Read the model definition and answer for the solid it produces. Units are mm, in the model's axes. Face numbers are marked on the shaded views. A direction names the side the tool comes from. Coordinates: 2 decimals unless noted, no trailing zeros. Order: outer loops, then holes, each group sorted by start corner. A loop starts at its lowest first (then second) coordinate and runs counter-clockwise, first axis right, second up. Notation, with made-up numbers: M -8,53 L 21,53 A33 cw 21,87 Z; hole C 34,70 d5. An arc over 180 degrees is marked long. One line per question, with ' | ' between items. Start each with the question number.
1) Consider probe 1 along Z at (x, y) = (2, 25); probe 2 along X at (y, z) = (18, 20.5); probe 3 along Y at (x, z) = (22.5, 63.75). Determine where each line is inside the solid, lowest interval first.
2) Find section D-D, the plane y = 4. Write down the section's boundary in (x, z), plus the area to 3 significant figures.
3) Find section A-A, the plane z = 40. Write down the section's boundary in (x, y), plus the area to 3 significant figures.
4) A tool of negligible diameter and unlimited length cuts with its end or side. For the marked faces 5, 6 and 7, from which of +Z, -Z, +X, -X, +Y, -Y can it reach the whole face along a straight path? Write none if from no direction.
5) Given P1, Ø23, axis at y = 25, z = 40, coming from the +X side; P2, Ø5, axis at x = 50.5, y = 32, coming from the +Z side; P3, Ø24, axis at x = 22.5, y = 25, coming from the -Z side, each flat-ended and moving along its own axis, determine where each tip first touches the part or whether it passes through.
6) The mould has two halves that part along X. Classify the marked faces 1, 2, 3 and 4: +X half, -X half, draft (parallel to the pull), parting line (faces both ways), or undercut.
7) Find section C-C, the plane y = 25. Count the separate pieces of the cut face and the enclosed holes in it, plus the area to 3 significant figures.
8) Find section B-B, the plane x = 22.5. Write down the section's boundary in (y, z), plus the area to 4 significant figures.
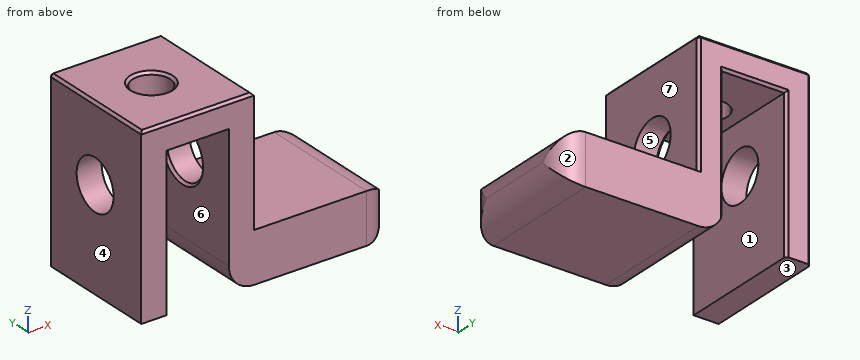
from build123d import *

# Parameters (mm, degrees)
F0_W     = 100
F0_H     = 50
F1_DEPTH = 20
F2_W     = 45
F2_H     = 50
F3_DEPTH = 50
F4_W     = 25
F4_H     = 60
F5_DEPTH = 50.001
F6_R     = 10
F7_DEPTH = 45
F8_R     = 7.5
F9_DEPTH = 70.001
F10_SIZE = 1
F11_R    = 9.99999


# Not quite as in the source:
# - a fillet or chamfer is up to 0.001 mm smaller than in the source, because OpenCascade refuses the exact size


with BuildPart() as f1:
    # F0 (on Top) → F1 (new body)
    with BuildSketch(Plane.XY):
        with Locations((50, 25)):
            Rectangle(F0_W, F0_H)
    extrude(amount=F1_DEPTH)

    # F2 (on face) → F3 (join)
    with BuildSketch(Plane.XY.offset(20)):
        with Locations((22.5, 25)):
            Rectangle(F2_W, F2_H)
    extrude(amount=F3_DEPTH)

    # F4 (on face) → F5 (cut, through all)
    with BuildSketch(Plane.XZ):
        with Locations((22.5, 30)):
            Rectangle(F4_W, F4_H)
    extrude(amount=-F5_DEPTH, mode=Mode.SUBTRACT)

    # F6 (on face) → F7 (cut, through all)
    with BuildSketch(Plane(origin=(0, 0, 0), x_dir=(0, -1, 0), z_dir=(-1, 0, 0))):
        with Locations((-25, 40)):
            Circle(F6_R)
    extrude(amount=-F7_DEPTH, mode=Mode.SUBTRACT)

    # F8 (on face) → F9 (cut, through all)
    with BuildSketch(Plane.XY.offset(70)):
        with Locations((22.5, 25)):
            Circle(F8_R)
    extrude(amount=-F9_DEPTH, mode=Mode.SUBTRACT)

    # F10
    f10_edges = [f1.edges().sort_by_distance(p)[0] for p in [
        (45, 50, 45),
        (22.5, 50, 70),
        (45, 25, 70),
        (0, 25, 70),
        (0, 50, 35),
        (10, 50, 30),
        (22.5, 50, 60),
        (35, 50, 30),
        (35, 35, 40),
        (15, 25, 70),
        (22.5, 0, 70),
    ]]
    chamfer(f10_edges, length=F10_SIZE)

    # F11 (radius 10 in the source; OpenCascade refuses exactly that, so slightly less here)
    f11_edges = [f1.edges().sort_by_distance(p)[0] for p in [
        (35, 24.5, 0),
        (100, 25, 0),
        (100, 0, 10),
        (100, 25, 20),
        (100, 50, 10),
    ]]
    fillet(f11_edges, radius=F11_R)


solid = f1.part
Report:
1) probe 1: z = 0 to 30, 50 to 70 | probe 2: x = 0 to 10, 35 to 45 | probe 3: y = 0 to 17.5, 32.5 to 50
2) outline: M 0,0 L 10,0 L 10,60 L 35,60 L 35,10 A10 ccw 45,0 L 90,0 A10 ccw 98,4 L 98,16 A10 ccw 90,20 L 45,20 L 45,69 L 44,70 L 1,70 L 0,69 Z | area: 2,670 mm^2
3) outline: M 0,0 L 10,0 L 10,15 L 0,15 Z; M 0,35 L 10,35 L 10,49 L 9,50 L 1,50 L 0,49 Z; M 35,0 L 45,0 L 45,15 L 36,15 L 35,14 Z; M 35,36 L 36,35 L 45,35 L 45,49 L 44,50 L 36,50 L 35,49 Z | area: 597 mm^2
4) face 5: +X, -X | face 6: -Z, +Y, -Y | face 7: +Z, +X, +Y, -Y
5) P1: stops at x = 45 | P2: stops at z = 20 | P3: stops at z = 60
6) face 1: undercut | face 2: +X half | face 3: draft | face 4: -X half
7) separate pieces: 4 | enclosed holes: 0 | area: 2,130 mm^2
8) outline: M 0,60 L 17.5,60 L 17.5,69 L 16.5,70 L 1,70 L 0,69 Z; M 32.5,60 L 49,60 L 50,61 L 50,69 L 49,70 L 33.5,70 L 32.5,69 Z | area: 347.5 mm^2
